Verification items for the finished model (mm, model axes). Coordinates: 2 decimals unless noted, no trailing zeros. Use a Markdown table: item, result. Add a question column.
from build123d import *

# Parameters (mm, degrees)
SKETCH2_W           = 90
SKETCH2_H           = 90
SKETCH1_W           = 200
SKETCH1_H           = 200
SKETCH6_W           = 210
SKETCH6_H           = 210
BOSS_EXTRUDE1_DEPTH = 5
SKETCH5_W           = 100
SKETCH5_H           = 100
BOSS_EXTRUDE2_DEPTH = 5
SKETCH3_W           = 80
SKETCH3_H           = 80
SKETCH4_W           = 190
SKETCH4_H           = 190


with BuildPart() as part:
    # Sketch2 → Loft2 section 0
    with BuildSketch(Plane.XY.offset(200)):
        Rectangle(SKETCH2_W, SKETCH2_H)
    # Sketch1 → Loft2 section 1
    with BuildSketch(Plane.XY):
        Rectangle(SKETCH1_W, SKETCH1_H)
    loft()

    # Sketch6 → Boss-Extrude1 (add)
    with BuildSketch(Plane(origin=(0, 0, 0), x_dir=(-1, 0, 0), z_dir=(0, 0, -1))):
        Rectangle(SKETCH6_W, SKETCH6_H)
    extrude(amount=-BOSS_EXTRUDE1_DEPTH)

    # Sketch5 → Boss-Extrude2 (add)
    with BuildSketch(Plane.XY.offset(200)):
        Rectangle(SKETCH5_W, SKETCH5_H)
    extrude(amount=-BOSS_EXTRUDE2_DEPTH)

    # Sketch3 → Cut-Loft2 section 0
    with BuildSketch(Plane.XY.offset(200)):
        Rectangle(SKETCH3_W, SKETCH3_H)
    # Sketch4 → Cut-Loft2 section 1
    with BuildSketch(Plane(origin=(0, 0, 0), x_dir=(-1, 0, 0), z_dir=(0, 0, -1))):
        Rectangle(SKETCH4_W, SKETCH4_H)
    loft(mode=Mode.SUBTRACT)


solid = part.part
1) Thickness scan on L1, parallel to X at y = -51.5, z = 68; L2, parallel to Y at x = 43.5, z = 22.5; L3, parallel to Y at x = -38, z = 173 (3 decimals). Record the ranges inside material, lowest first.
2) Release check for a two-part mould opening along Z. For faces 1 (the face through (-4, -48, 195)), 2 (the face through (8, -101, 0)), 3 (the face through (8, -101, 5)) record: released by +Z, released by -Z, zero draft, split by the parting line, or undercut.
3) Gauge pin test, flat ends, axial feed: pin 1 (12 mm diameter, centred on y = -60.5, z = 111.5, fed in from +X); pin 2 (12 mm diameter, centred on x = -16, z = 161.5, fed in from +Y); pin 3 (4 mm diameter, centred on x = 6, z = 197.5, fed in from +Y). Record the tip position at first contact, or that the pin passes through.
Returned:
| question | item | result |
|---|---|---|
| 1 | L1 | x = -81.3 to -76.3, 76.3 to 81.3 |
| 1 | L2 | y = -93.81 to -88.81, 88.81 to 93.81 |
| 1 | L3 | y = -52.425 to -47.425, 47.425 to 52.425 |
| 2 | face 1 | undercut |
| 2 | face 2 | released by -Z |
| 2 | face 3 | released by +Z |
| 3 | pin 1 | stops at x = 70.99 |
| 3 | pin 2 | stops at y = 57.24 |
| 3 | pin 3 | stops at y = 50 |
